```python
from build123d import *

# Parameters (mm, degrees)
ESQUISSE1_R             = 2
BOSS_EXTRU_1_DEPTH      = 5
ESQUISSE2_R             = 1.5
ESQUISSE2_R_2           = 1
BOSS_EXTRU_2_DEPTH      = 2
BOSS_EXTRU_3_START      = 3
ESQUISSE3_R             = 1
ESQUISSE3_R_2           = 0.5
BOSS_EXTRU_3_DEPTH      = 3
CONG_1_R                = 0.5
CONG_2_R                = 0.5
ESQUISSE5_R             = 0.5
ENL_V_MAT_EXTRU_1_DEPTH = 2


with BuildPart() as part:
    # Esquisse1 → Boss.-Extru.1 (new body)
    with BuildSketch(Plane.XY):
        Circle(ESQUISSE1_R)
    extrude(amount=BOSS_EXTRU_1_DEPTH)

    # Esquisse2 → Boss.-Extru.2 (add)
    with BuildSketch(Plane.XY.offset(5)):
        Circle(ESQUISSE2_R)
        Circle(ESQUISSE2_R_2, mode=Mode.SUBTRACT)
    extrude(amount=BOSS_EXTRU_2_DEPTH)

    # Esquisse3 → Boss.-Extru.3 (add)
    with BuildSketch(Plane(origin=(0, 0, 0), x_dir=(-1, 0, 0), z_dir=(0, 0, -1)).offset(BOSS_EXTRU_3_START)):
        with Locations(Location((0, 0, 0), (0, 0, 180))):
            Circle(ESQUISSE3_R)
        Circle(ESQUISSE3_R_2, mode=Mode.SUBTRACT)
    extrude(amount=-BOSS_EXTRU_3_DEPTH)

    # Congé1
    cong_1_edges = [part.edges().sort_by_distance(p)[0] for p in [
        (-1, 0, 0),
    ]]
    fillet(cong_1_edges, radius=CONG_1_R)

    # Congé2
    cong_2_edges = [part.edges().sort_by_distance(p)[0] for p in [
        (-1.5, 0, 5),
    ]]
    fillet(cong_2_edges, radius=CONG_2_R - 0.0001)  # a hair under: the kernel refuses the full size

    # Esquisse5 → Enlèv. mat.-Extru.1 (cut)
    with BuildSketch(Plane(origin=(0, 0, 0), x_dir=(1, 0, 0), z_dir=(0, 1, 0))):
        with Locations(Location((0, 1.75, 0), (0, 0, 270))):
            Circle(ESQUISSE5_R)
        with Locations(Location((0, -6.25, 0), (0, 0, 270))):
            Circle(ESQUISSE5_R)
    extrude(amount=-ENL_V_MAT_EXTRU_1_DEPTH, mode=Mode.SUBTRACT)


solid = part.part
```
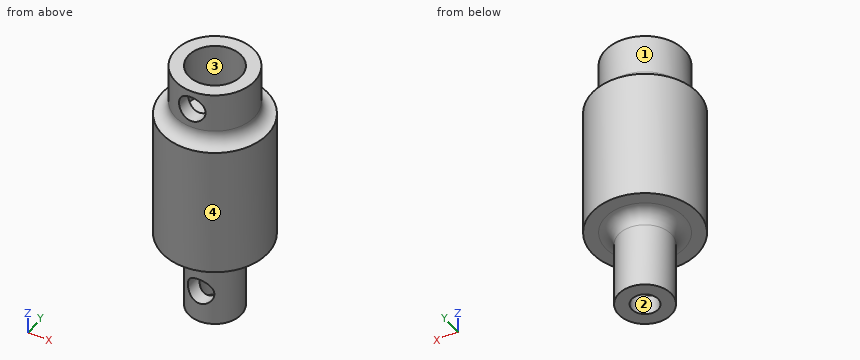
Geometry: final body of the model. Coordinates: model frame, mm. Face numbers are marked on the shaded views. A direction names the side the tool comes from. Coordinates: 2 decimals unless noted, no trailing zeros. Loops run counter-clockwise (first coordinate to the right, second up) from the corner with the lowest first, then second, coordinate; pieces in that order, holes last. Notation, with made-up numbers: (19, 5.25) -> (29, 5.25) arc R14 cw to (29, 32.25) -> close; hole circle Ø9 at (0, -20.5). An arc over 180 degrees is marked (long way). Use a Markdown table: item, result. Add a question column.
(1) Mould query, pull axis X, two halves, no side actions, for the marked faces 3 and 4. Classes: pulls with the +X half, pulls with the -X half, needs draft (parallel to the pull), parting line crosses it, or undercut.
(2) Pin query (flat end, axial travel): pin 1 Ø1.5 at (x, y) = (-0.5, -1) entering from -Z; pin 2 Ø1.6 at (x, y) = (0, 0) entering from +Z; pin 3 Ø0.8 at (x, y) = (0, 0) entering from -Z. Return the tip coordinate at first contact, or that it passes through.
(3) Section query A-A, the plane x = 0. State how many separate pieces and enclosed holes the cut face has, plus the area to 3 significant figures.
(4) Line query: line 1 along Y through (x, z) = (0, 5.6); line 2 along Y through (x, z) = (0, -2.4); line 3 along Y through (x, z) = (0, -2.1). Output: solid intervals per line, ascending.
(5) Section query B-B, the plane z = 1.25. Return loops of the section in (x, y), plus the area to 3 significant figures.
(6) Section query D-D, the plane z = -1.75. Return loops of the section in (x, y), plus the area to 3 significant figures.
(7) Section query C-C, the plane z = 6.5. Return loops of the section in (x, y), plus the area to 3 significant figures.
(8) Access query for the marked faces 1 and 2. Directions: +Z, -Z, +X, -X, +Y, -Y. A direction counts if a zero-diameter tool reaches every point of the face in a straight line with its end or side. Return the directions, or none.
Answer:
| question | item | result |
|---|---|---|
| 1 | face 3 | undercut |
| 1 | face 4 | parting line crosses it |
| 2 | pin 1 | stops at z = -3 |
| 2 | pin 2 | stops at z = 5 |
| 2 | pin 3 | stops at z = 0 |
| 3 | separate pieces | 3 |
| 3 | enclosed holes | 0 |
| 3 | area | 24.2 mm^2 |
| 4 | line 1 | y = -1.5 to -1, 1 to 1.5 |
| 4 | line 2 | y = -1 to -0.5, 0.5 to 1 |
| 4 | line 3 | y = 0.5 to 1 |
| 5 | outline | circle Ø4 at (0, 0) |
| 5 | area | 12.6 mm^2 |
| 6 | outline | (-0.5, -0.87) -> (-0.5, 0) arc R0.5 cw to (0.5, 0) -> (0.5, -0.87) arc R1 ccw (long way) to start |
| 6 | area | 1.79 mm^2 |
| 7 | outline | (-0.43, -1.44) -> (-0.43, -0.9) arc R1 cw (long way) to (0.43, -0.9) -> (0.43, -1.44) arc R1.5 ccw (long way) to start |
| 7 | area | 3.48 mm^2 |
| 8 | face 1 | +Z |
| 8 | face 2 | -Z |
